Answer from the drawing. Dimensions are ordinates in mm from the lowest x, y and z of the part. A direction names the side the tool comes from. Coordinates: 2 decimals unless noted, no trailing zeros. Loops run counter-clockwise (first coordinate to the right, second up) from the corner with the lowest first, then second, coordinate; pieces in that order, holes last. Notation, with made-up numbers: M 33.5,11 L 46.5,11 A9 cw 46.5,16 Z; hole C 32,59.25 d8. An arc over 180 degrees is marked long. One line per item, written item: value. Start each with the question number.
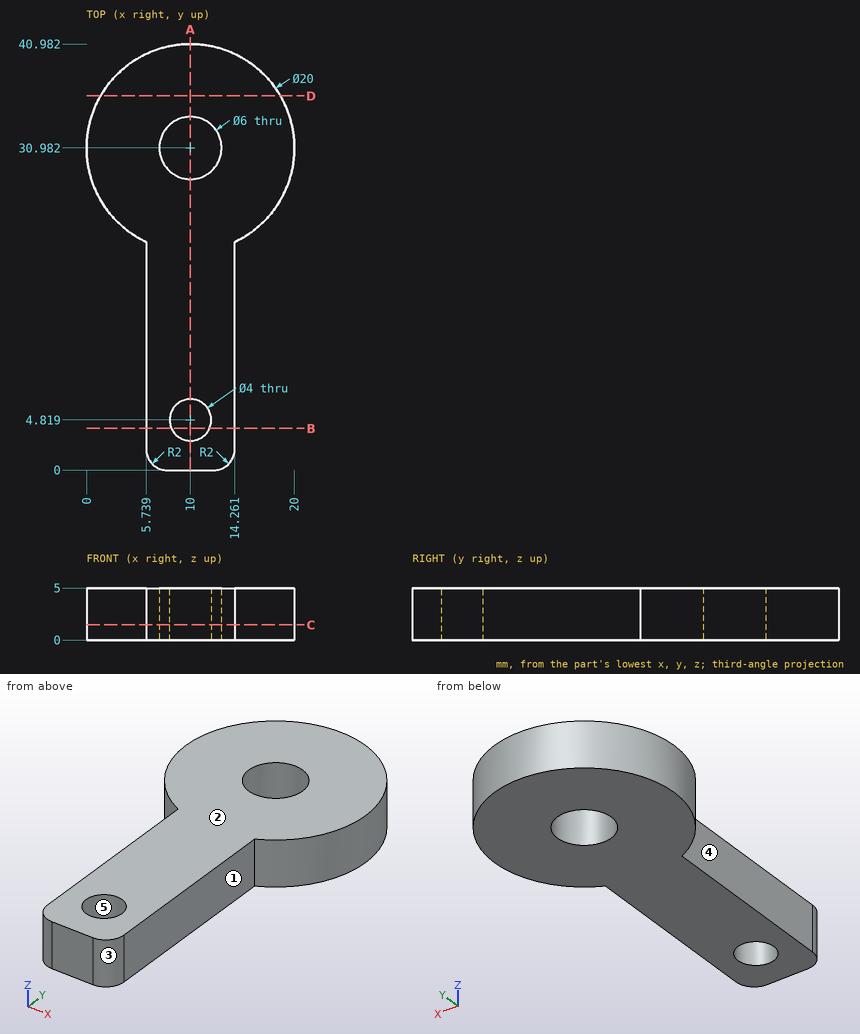
1) For a pull along Y with two mould halves and no side action, classify the marked faces 3, 4 and 5 as released by +Y, released by -Y, zero draft, split by the parting line, or undercut.
2) Section A-A (x = 10) is taken. Determine the outline of the cut face in (y, z).
3) Section B-B (y = 4) is taken. Determine the outline of the cut face in (x, z) (1 decimal).
4) Section D-D (y = 36) is taken. Determine the outline of the cut face in (x, z).
5) A tool of negligible diameter and unlimited length cuts with its end or side. For the marked faces 1 and 2, from which of +Z, -Z, +X, -X, +Y, -Y can it reach the whole face along a straight path? Write none if from no direction.
6) Section C-C (z = 1.45) is taken. Determine the outline of the cut face in (x, y) (1 decimal).
7) Flat-ended cylindrical pins translate along their axes: pin 1 (1.5 mm diameter, centred on y = 12.5, z = 3.5, fed in from -X); pin 2 (1.5 mm diameter, centred on y = 13.5, z = 2.5, fed in from +X); pin 3 (2 mm diameter, centred on x = 15.5, z = 3, fed in from -Y). Find the tip coordinate at first contact, or state that the pin passes through.
8) Consider line 1 along Y through (x, z) = (10, 2.85); line 2 along X through (y, z) = (5, 4.05); line 3 along Y through (x, z) = (9.5, 1.3) (1 decimal). Determine where each line is inside the solid, lowest interval first.
Results found:
1. face 3: released by -Y
1. face 4: zero draft
1. face 5: undercut
2. outline: M 0,0 L 2.82,0 L 2.82,5 L 0,5 Z; M 6.82,0 L 27.98,0 L 27.98,5 L 6.82,5 Z; M 33.98,0 L 40.98,0 L 40.98,5 L 33.98,5 Z
3. outline: M 5.7,0 L 8.2,0 L 8.2,5 L 5.7,5 Z; M 11.8,0 L 14.3,0 L 14.3,5 L 11.8,5 Z
4. outline: M 1.35,0 L 18.65,0 L 18.65,5 L 1.35,5 Z
5. face 1: +Z, -Z, +X, -Y
5. face 2: +Z, +X, -X, +Y, -Y
6. outline: M 5.7,2 A2 ccw 7.7,0 L 12.3,0 A2 ccw 14.3,2 L 14.3,21.9 A10 ccw long 5.7,21.9 Z; hole C 10,31 d6; hole C 10,4.8 d4
7. pin 1: stops at x = 5.74
7. pin 2: stops at x = 14.26
7. pin 3: stops at y = 22.05
8. line 1: y = 0 to 2.82, 6.82 to 27.98, 33.98 to 40.98
8. line 2: x = 5.74 to 8.01, 11.99 to 14.26
8. line 3: y = 0 to 2.9, 6.8 to 28, 33.9 to 41
